from build123d import *

# Parameters (mm, degrees)
F2_R     = 4.7625
F3_DEPTH = 8
F4_R     = 4.7625
F5_DEPTH = 6


with BuildPart() as f1:
    # F0 (on Front) → F1 (revolve)
    with BuildSketch(Plane.XZ):
        Polygon((-13.4615, 0), (-4.7625, 0), (-4.7625, 35), (-9.4615, 35), (-9.4615, 10.5), (-13.4615, 10.5), (-13.4615, 17.1237489689), (-17.25, 10.5618744845), (-17.25, 6.5618744845), align=None)
    revolve(axis=Axis((0, 0, 27.3268250281), (0, 0, 1)))

    # F2 (on face) → F3 (cut)
    with BuildSketch(Plane.XY.offset(35)):
        Polygon((3.897114317, 6.75), (-3.897114317, 6.75), (-7.7942286341, 0), (-3.897114317, -6.75), (3.897114317, -6.75), (7.7942286341, 0), align=None)
        Circle(F2_R, mode=Mode.SUBTRACT)
    extrude(amount=-F3_DEPTH, mode=Mode.SUBTRACT)

    # F4 (on face) → F5 (cut)
    with BuildSketch(Plane(origin=(0, 0, 0), x_dir=(1, 0, 0), z_dir=(0, 0, -1))):
        Polygon((3.897114317, 6.75), (-3.897114317, 6.75), (-7.7942286341, 0), (-3.897114317, -6.75), (3.897114317, -6.75), (7.7942286341, 0), align=None)
        Circle(F4_R, mode=Mode.SUBTRACT)
    extrude(amount=-F5_DEPTH, mode=Mode.SUBTRACT)


solid = f1.part
CAD build for the part. Positions are in the model's coordinates, mm. A direction names the side the tool comes from. Give positions to 0.01 mm unless a question says otherwise; leave off trailing zeros. Order: outer loops, then holes, each group sorted by start corner. A loop starts at its lowest first (then second) coordinate and runs counter-clockwise, first axis right, second up. Notation, with made-up numbers: (4, 75.5) -> (23, 75.5) arc R37 ccw to (23, 111.5) -> close; hole circle Ø1 at (-5.75, 32.25). An arc over 180 degrees is marked (long way). Return JSON: item names as keys, results as strings.
Q1. Saw through at B-B (x = 0). Write the cut outline in (y, z), then the cut area to 3 significant figures.
Working result:
{"outline": "(-17.25, 6.56) -> (-13.46, 0) -> (-6.75, 0) -> (-6.75, 6) -> (-4.76, 6) -> (-4.76, 27) -> (-6.75, 27) -> (-6.75, 35) -> (-9.46, 35) -> (-9.46, 10.5) -> (-13.46, 10.5) -> (-13.46, 17.12) -> (-17.25, 10.56) -> close; (4.76, 6) -> (6.75, 6) -> (6.75, 0) -> (13.46, 0) -> (17.25, 6.56) -> (17.25, 10.56) -> (13.46, 17.12) -> (13.46, 10.5) -> (9.46, 10.5) -> (9.46, 35) -> (6.75, 35) -> (6.75, 27) -> (4.76, 27) -> close", "area": "437 mm²"}
Q2. Saw through at D-D (z = 24.5). Write the cut outline in (x, y) (1 decimal), then the cut area to 3 significant figures.
Working result:
{"outline": "circle Ø18.9 at (0, 0); hole circle Ø9.5 at (0, 0)", "area": "210 mm²"}
Q3. Saw through at C-C (z = 15.5). Write the cut outline in (x, y) (1 decimal).
Working result:
{"outline": "circle Ø28.8 at (0, 0); circle Ø18.9 at (0, 0); hole circle Ø26.9 at (0, 0); hole circle Ø9.5 at (0, 0)"}
Q4. Flat gauge pins, fed straight in: pin 1 (10 mm diameter, centred on y = -7.5, z = 11.5, fed in from -X); pin 2 (12.5 mm diameter, centred on x = 0, y = 0, fed in from +Z); pin 3 (8 mm diameter, centred on x = -5.5, z = 13.5, fed in from -Y). Where does each tip first touch, or does it go through?
Working result:
{"pin 1": "x = -17.05", "pin 2": "z = 27", "pin 3": "y = -17.02"}
Q5. Mould opens along X. For faces 4 (the face through (0, 6.75, 3)), 5 (the face through (-13.015, -4.099, 0.319)), 6 (the face through (-6.4, 2.8, 35)) say: pulls with the +X half, pulls with the -X half, needs draft (parallel to the pull), parting line crosses it, or undercut.
Working result:
{"face 4": "undercut", "face 5": "parting line crosses it", "face 6": "needs draft"}
Q6. Saw through at A-A (z = 32.5). Write the cut outline in (x, y), then the cut area to 3 significant figures.
Working result:
{"outline": "circle Ø18.92 at (0, 0); hole (-7.79, 0) -> (-3.9, -6.75) -> (3.9, -6.75) -> (7.79, 0) -> (3.9, 6.75) -> (-3.9, 6.75) -> close", "area": "123 mm²"}
Q7. Which spindle directions (+Z, -Z, +X, -X, +Y, -Y) get a long thin tool onto all of the face, cutting with end or side? Do faces 1 (the face through (2, 5, 27)), 2 (the face through (-5.87, 3.33, 2.96)), 3 (the face through (-16.453, -5.181, 8.534)). Say none if no direction does.
Working result:
{"face 1": "+Z", "face 2": "-Z", "face 3": "+Z, -Z"}
Q8. Drill centre lines: line 1 (Y direction, x = 0, z = 12); line 2 (X direction, y = 0, z = 13.75); line 3 (Y direction, x = 8.5, z = 15.5). Where is each one in solid material? Low to high.
Working result:
{"line 1": "-16.42 to -13.46, -9.46 to -4.76, 4.76 to 9.46, 13.46 to 16.42", "line 2": "-15.41 to -13.46, -9.46 to -4.76, 4.76 to 9.46, 13.46 to 15.41", "line 3": "-11.62 to -10.44, -4.16 to 4.16, 10.44 to 11.62"}
